Input: part model. Units: mm. Frame: model coordinates. Face numbers are marked on the shaded views. A direction names the side the tool comes from. Give positions to 0.01 mm unless a question says otherwise; leave off trailing zeros. Write each loop counter-clockwise with the first axis right and the second up, starting at its lowest first coordinate (ties: lowest second). Pieces come first, ordered by that corner, then holes. Notation, with made-up numbers: (89.25, -11.75) -> (139.25, -11.75) arc R25 cw to (139.25, 6.25) -> close; hole circle Ø4 at (66, 56.25). An arc over 180 degrees is marked (long way). Return JSON: item names as keys, results as strings. Group by question number.
Item 1: Section A-A, the plane x = -6. Return loops of the section in (y, z), then the cut area to 3 significant figures.
Item 2: Line query: line 1 (X direction, y = 10.25, z = -12); line 2 (X direction, y = 10.5, z = -3); line 3 (X direction, y = 7.75, z = 4). Output: solid intervals per line, ascending. Write a range as [from, to].
Item 3: Set-up query: the marked faces 1, 2 and 3. Return all of +Z, -Z, +X, -X, +Y, -Y with unobstructed straight access to the full face (end or side cutting, diameter ignored); none if empty.
Item 4: Mould query, pull axis X, two halves, no side actions, for the marked faces 4, 5, 6 and 7. Classes: released by +X, released by -X, zero draft, split by the parting line, or undercut.
Item 5: Pin query (flat end, axial travel): P1, Ø4, axis at x = 0.5, z = -2.5, coming from the +Y side; P2, Ø1, axis at x = 14, z = -8.5, coming from the +Y side; P3, Ø9, axis at x = 2, z = 3, coming from the +Y side. Return the tip coordinate at first contact, or that it passes through.
Item 6: Section B-B, the plane z = 13. Return loops of the section in (x, y), then the cut area to 3 significant figures.
Item 7: Section C-C, the plane y = 6.25. Return loops of the section in (x, z).
Item 8: Section D-D, the plane x = 1. Return loops of the section in (y, z), then the cut area to 3 significant figures.
from build123d import *

# Parameters (mm, degrees)
SKETCH_1_W           = 30
SKETCH_1_H           = 40
EXTRUDE_1_DEPTH      = 8
CHAMFER_1_SIZE       = 5
CHAMFER_1_SIZE2      = 2.886751346
EXTRUDE_START        = -3
EXTRUDE_2_DEPTH      = 3.5
EXTRUDE_3_DEPTH      = 10
EXTRUDE_3_DEPTH_BACK = 10
SKETCH_4_W           = 4
SKETCH_4_H           = 4
CUT_EXTRUDE_2_DEPTH  = 1
SKETCH_12_W          = 10
SKETCH_12_H          = 12
CUT_EXTRUDE_3_DEPTH  = 1


with BuildPart() as part:
    # 草图1 → 凸台-拉伸1 (new body)
    with BuildSketch(Plane(origin=(0, 0, 0), x_dir=(1, 0, 0), z_dir=(0, 1, 0))):
        Rectangle(SKETCH_1_W, SKETCH_1_H)
    extrude(amount=EXTRUDE_1_DEPTH)

    # 倒角1
    chamfer_1_edges = [part.edges().sort_by_distance(p)[0] for p in [
        (0, 8, 20),
    ]]
    chamfer_1_side = [part.faces().sort_by_distance(p)[0] for p in [
        (0, 4, 20),
    ]]
    chamfer(chamfer_1_edges, length=CHAMFER_1_SIZE, length2=CHAMFER_1_SIZE2, reference=chamfer_1_side[0])

    # 草图6 → 凸台-拉伸2 (add)
    with BuildSketch(Plane(origin=(15, 0, 0), x_dir=(0, 0, -1), z_dir=(1, 0, 0)).offset(EXTRUDE_START)):
        with BuildLine():
            Line((18, 12), (18, 4))
            ThreePointArc((18, 4), (17.707106781, 3.292893219), (17, 3))
            Line((17, 3), (-1, 3))
            ThreePointArc((-1, 3), (-1.707106781, 3.292893219), (-2, 4))
            Line((-2, 4), (-2, 12))
            ThreePointArc((-2, 12), (-1.707106781, 12.707106781), (-1, 13))
            Line((-1, 13), (17, 13))
            ThreePointArc((17, 13), (17.707106781, 12.707106781), (18, 12))
        make_face()
    extrude_2 = extrude(amount=EXTRUDE_2_DEPTH)

    # 镜向2: 凸台-拉伸2 across plane
    add(extrude_2.mirror(Plane(origin=(0, 0, 0), x_dir=(0, 0, 1), z_dir=(1, 0, 0))))

    # 草图10 → 凸台-拉伸3 (add, two sides: drawn at the far end of the back side and taken through both)
    with BuildSketch(Plane(origin=(0, 0, 0), x_dir=(0, 0, -1), z_dir=(1, 0, 0)).offset(-EXTRUDE_3_DEPTH_BACK)):
        with BuildLine():
            Line((9, 8), (9, 15.630981347))
            ThreePointArc((9, 15.630981347), (10.780355092, 17.991396878), (12.965661526, 16))
            Line((12.965661526, 16), (12.965661526, 8))
            Line((12.965661526, 8), (9, 8))
        make_face()
    extrude(amount=EXTRUDE_3_DEPTH + EXTRUDE_3_DEPTH_BACK)

    # 草图4 → 切除-拉伸2 (cut)
    with BuildSketch(Plane(origin=(0, 8, 0), x_dir=(1, 0, 0), z_dir=(0, 1, 0))):
        with Locations((-10, -12)):
            Rectangle(SKETCH_4_W, SKETCH_4_H)
        with Locations((10, -12)):
            Rectangle(SKETCH_4_W, SKETCH_4_H)
    extrude(amount=-CUT_EXTRUDE_2_DEPTH, mode=Mode.SUBTRACT)

    # 草图12 → 切除-拉伸3 (cut)
    with BuildSketch(Plane(origin=(0, 8, 0), x_dir=(1, 0, 0), z_dir=(0, 1, 0))):
        with Locations((0, -8)):
            Rectangle(SKETCH_12_W, SKETCH_12_H)
    extrude(amount=-CUT_EXTRUDE_3_DEPTH, mode=Mode.SUBTRACT)

    # 草图14 → 放样3 section 0
    with BuildSketch(Plane(origin=(0, 12, 0), x_dir=(1, 0, 0), z_dir=(0, 1, 0))):
        with BuildLine():
            Line((-4.5, -7.020034464), (4.5, -7.020034464))
            Line((4.5, -7.020034464), (4.5, -9.020034464))
            Line((4.5, -9.020034464), (-4.5, -9.020034464))
            Line((-4.5, -9.020034464), (-4.5, -7.020034464))
        make_face()
    # 草图13 → 放样3 section 1
    with BuildSketch(Plane(origin=(0, 7, 0), x_dir=(1, 0, 0), z_dir=(0, 1, 0))):
        with BuildLine():
            Line((-4.5, -10), (4.5, -10))
            Line((4.5, -10), (4.5, -6))
            Line((4.5, -6), (-4.5, -6))
            Line((-4.5, -6), (-4.5, -10))
        make_face()
    loft()


solid = part.part
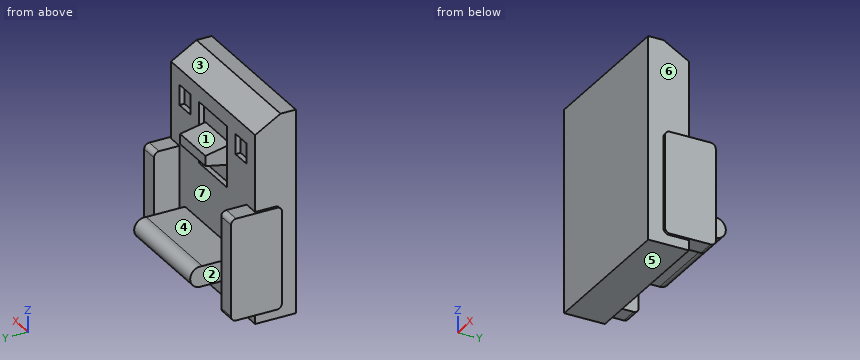
Answer below:
{
 "1": {"outline": "(0, -20) -> (8, -20) -> (8, -12.97) -> (16, -12.97) arc R2 ccw (long way) to (15.63, -9) -> (8, -9) -> (8, 17.11) -> (3, 20) -> (0, 20) -> close", "area": "351 mm2"},
 "2": {"line 1": "x = [-15.5, -12], [-10, 10], [12, 15.5]", "line 2": "x = [-15.5, -12], [12, 15.5]", "line 3": "x = [-15, -5], [5, 15]"},
 "3": {"face 1": "+Y", "face 2": "+Z, -Z, +Y", "face 3": "+Z, +X, -X, +Y"},
 "4": {"face 4": "undercut", "face 5": "zero draft", "face 6": "released by +X", "face 7": "undercut"},
 "5": {"P1": "stops at y = 8", "P2": "stops at y = 13", "P3": "stops at y = 12"},
 "6": {"outline": "(-15, 0) -> (15, 0) -> (15, 8) -> (12, 8) -> (12, 7) -> (8, 7) -> (8, 8) -> (5, 8) -> (5, 7) -> (-5, 7) -> (-5, 8) -> (-8, 8) -> (-8, 7) -> (-12, 7) -> (-12, 8) -> (-15, 8) -> close", "area": "222 mm2"},
 "7": {"outline": "(-15.5, -18) -> (-15, -18) -> (-15, -20) -> (15, -20) -> (15, -18) -> (15.5, -18) -> (15.5, 2) -> (15, 2) -> (15, 18.12) -> (-15, 18.12) -> (-15, 2) -> (-15.5, 2) -> close"},
 "8": {"outline": "(0, -20) -> (8, -20) -> (8, -12.97) -> (16, -12.97) arc R2 ccw (long way) to (15.63, -9) -> (8, -9) -> (8, 2) -> (7, 2) -> (7, 6) -> (12, 7.02) -> (12, 9.02) -> (7, 10) -> (7, 14) -> (8, 14) -> (8, 17.11) -> (3, 20) -> (0, 20) -> close", "area": "354 mm2"}
}
